Autodesk Inventor part; units mm, degrees
ref_plane "YZ Plane" through (0, 0, 0) normal (1, 0, 0) x (0, 1, 0)
ref_plane "XZ Plane" through (0, 0, 0) normal (0, 1, 0) x (-1, 0, 0)
ref_plane "XY Plane" through (0, 0, 0) normal (0, 0, 1) x (1, 0, 0)
sketch "Sketch5" plane through (0, 0, 0) normal (0, 0, 1) x (1, 0, 0)
  line L0 (-31, 52.5) -> (31, 52.5)
  line L1 (31, 52.5) -> (31, -52.5)
  line L2 (-31, -52.5) -> (-31, 52.5)
  line L3 (-15.5, 27.5) -> (-15.5, -52.5) construction
  line L4 (-18.25, 27.5) -> (-18.25, -52.5)
  line L5 (-12.75, -52.5) -> (-12.75, 27.5)
  arc A0 (-12.75, 27.5) -> (-18.25, 27.5) centre (-15.5, 27.5) ccw
  arc A1 (-18.25, -52.5) -> (-12.75, -52.5) centre (-15.5, -52.5) ccw
  line L6 (0, 0) -> (0, 14.7878) construction
  line L7 (15.5, 27.5) -> (15.5, -52.5) construction
  line L8 (18.25, 27.5) -> (18.25, -52.5)
  line L9 (12.75, -52.5) -> (12.75, 27.5)
  arc A2 (18.25, 27.5) -> (12.75, 27.5) centre (15.5, 27.5) ccw
  arc A3 (12.75, -52.5) -> (18.25, -52.5) centre (15.5, -52.5) ccw
  line L10 (-18.25, -52.5) -> (-31, -52.5)
  line L11 (31, -52.5) -> (18.25, -52.5)
  line L12 (12.75, -52.5) -> (-12.75, -52.5)
  point P0 (0, 52.5)
  point P1 (-31, 0)
  point P2 (-15.5, -12.5)
  dimension "d8" = 62
  dimension "d9" = 105
  dimension "d10" = 15.5
  dimension "d11" = 5.5
  dimension "d12" = 80
extrude "Extrusion5" add sketch "Sketch5" along normal blind 2.6 contours L0 L1 L11 L8 A2 L9 L12 L5 A0 L4 L10 L2
chamfer "Chamfer1" distance 2 angle 45 8 edges at (-18.25, -52.5, 1.3) (-12.75, -52.5, 1.3) (12.75, -52.5, 1.3) (18.25, -52.5, 1.3) (31, -52.5, 1.3) (-31, -52.5, 1.3) (31, 52.5, 1.3) (-31, 52.5, 1.3)
sketch "Sketch6" plane through (0, 0, 2.6) normal (0, 0, 1) x (1, 0, 0)
  line L0 (29, 52.5) -> (-29, 52.5)
  line L1 (6, 49.5) -> (-6, 49.5) construction
  line L2 (6, 51) -> (-6, 51)
  line L3 (-6, 48) -> (6, 48)
  arc A0 (6, 48) -> (6, 51) centre (6, 49.5) ccw
  arc A1 (-6, 51) -> (-6, 48) centre (-6, 49.5) ccw
  point P0 (0, 0)
  point P1 (0, 49.5)
  dimension "d18" = 12
  dimension "d19" = 3
  dimension "d20" = 1.5
extrude "Extrusion6" cut sketch "Sketch6" against normal through all
properties part number "BC-10027" material "Aço Inox AISI 316"
Source: CAD feature listing. Evaluate the final solid. Frame: model axes, mm. A direction names the side the tool comes from. Round coordinates to 2 decimals unless told otherwise and drop trailing zeros. Loops run counter-clockwise (first coordinate to the right, second up) from the corner with the lowest first, then second, coordinate; pieces in that order, holes last.
1. Section query D-D on y = 49.5. Output: boundary loops of the cut face in (x, z).
2. Section query C-C on z = 1.3. Output: boundary loops of the cut face in (x, y).
3. Section query A-A on x = -0.5. Output: boundary loops of the cut face in (y, z), and give its area (3 significant figures).
4. Access query for faces 1 (the flat face through (-11.76, -51.49, 1.28)), 2 (the flat face through (0, 51, 1)), 3 (the flat face through (30, 51.5, 1.3)). Directions: +Z, -Z, +X, -X, +Y, -Y. A direction counts if a zero-diameter tool reaches every point of the face in a straight line with its end or side. Return the directions, or none.
5. Ray query, L1, parallel to X at y = -35.5, z = 2.1; L2, parallel to Y at x = -2, z = 2.4; L3, parallel to X at y = 30, z = 1.9. Return the intervals inside material, ascending.
6. Section query B-B on y = -43. Output: boundary loops of the cut face in (x, z), and give its area (3 significant figures).
7. Mould query, pull axis X, two halves, no side actions, for faces 4 (the flat face through (12.75, -12, 1)), 5 (the flat face through (0, -52.5, 1)), 6 (the flat face through (31, 1, 1)), 7 (the flat face through (-31, -1, 1)). Classes: released by +X, released by -X, zero draft, split by the parting line, or undercut.
Answers below:
1. outline: (-31, 0) - (-7.5, 0) - (-7.5, 2.6) - (-31, 2.6) - close; (7.5, 0) - (31, 0) - (31, 2.6) - (7.5, 2.6) - close
2. outline: (-31, -50.5) - (-29, -52.5) - (-20.25, -52.5) - (-18.25, -50.5) - (-18.25, 27.5) arc R2.75 cw to (-12.75, 27.5) - (-12.75, -50.5) - (-10.75, -52.5) - (10.75, -52.5) - (12.75, -50.5) - (12.75, 27.5) arc R2.75 cw to (18.25, 27.5) - (18.25, -50.5) - (20.25, -52.5) - (29, -52.5) - (31, -50.5) - (31, 50.5) - (29, 52.5) - (-29, 52.5) - (-31, 50.5) - close; hole (-6, 48) - (6, 48) arc R1.5 ccw to (6, 51) - (-6, 51) arc R1.5 ccw to start
3. outline: (-52.5, 0) - (48, 0) - (48, 2.6) - (-52.5, 2.6) - close; (51, 0) - (52.5, 0) - (52.5, 2.6) - (51, 2.6) - close
3. area: 265 mm2
4. face 1: +Z, -Z, -Y
4. face 2: +Z, -Z
4. face 3: +Z, -Z, +X, +Y
5. L1: x = -31 to -18.25, -12.75 to 12.75, 18.25 to 31
5. L2: y = -52.5 to 48, 51 to 52.5
5. L3: x = -31 to -16.65, -14.35 to 14.35, 16.65 to 31
6. outline: (-31, 0) - (-18.25, 0) - (-18.25, 2.6) - (-31, 2.6) - close; (-12.75, 0) - (12.75, 0) - (12.75, 2.6) - (-12.75, 2.6) - close; (18.25, 0) - (31, 0) - (31, 2.6) - (18.25, 2.6) - close
6. area: 133 mm2
7. face 4: undercut
7. face 5: zero draft
7. face 6: released by +X
7. face 7: released by -X
